```python
from build123d import *

# Parameters (mm, degrees)
SKETCH_1_W          = 8.99
SKETCH_1_H          = 1.99
EXTRUDE_1_DEPTH     = 1
EXTRUDE_2_DEPTH     = 8.99
SKETCH_3_W          = 1.62690844
SKETCH_3_H          = 0.234992706
CUT_EXTRUDE_2_DEPTH = 8.9
SKETCH_4_W          = 5.293711796
SKETCH_4_H          = 1.344910324
EXTRUDE_3_DEPTH     = 0.5
SKETCH_5_W          = 4.74668983
SKETCH_5_H          = 1.99
EXTRUDE_4_DEPTH     = 0.5
CHAMFER_1_SIZE      = 0.1
CHAMFER_2_SIZE      = 0.1


with BuildPart() as part:
    # 草图1 → 凸台-拉伸1 (new body)
    with BuildSketch(Plane(origin=(0, 0, 0), x_dir=(1, 0, 0), z_dir=(0, 1, 0))):
        Rectangle(SKETCH_1_W, SKETCH_1_H)
    extrude(amount=EXTRUDE_1_DEPTH)

    # 草图2 → 凸台-拉伸2 (add)
    with BuildSketch(Plane(origin=(4.495, 0, 0), x_dir=(0, 0, -1), z_dir=(1, 0, 0))):
        Polygon((-0.995, 0.5), (-1.355023595, 0.5), (-0.995, 1), align=None)
    extrude(amount=-EXTRUDE_2_DEPTH)

    # 草图3 → 切除-拉伸2 (cut)
    with BuildSketch(Plane(origin=(4.495, 0, 0), x_dir=(0, 0, -1), z_dir=(1, 0, 0))):
        with Locations((0, 0.75)):
            Rectangle(SKETCH_3_W, SKETCH_3_H)
    extrude(amount=-CUT_EXTRUDE_2_DEPTH, mode=Mode.SUBTRACT)

    # 草图4 → 凸台-拉伸3 (add)
    with BuildSketch(Plane.XZ):
        Rectangle(SKETCH_4_W, SKETCH_4_H)
    extrude(amount=EXTRUDE_3_DEPTH)

    # 草图5 → 凸台-拉伸4 (add)
    with BuildSketch(Plane(origin=(0, 1, 0), x_dir=(1, 0, 0), z_dir=(0, 1, 0))):
        Rectangle(SKETCH_5_W, SKETCH_5_H)
    extrude(amount=-EXTRUDE_4_DEPTH)

    # 倒角1
    chamfer_1_edges = [part.edges().sort_by_distance(p)[0] for p in [
        (2.646855898, 0, 0),
        (0, 0, 0.672455162),
        (-2.646855898, 0, 0),
        (0, 0, -0.672455162),
        (2.646855898, -0.5, 0),
        (0, -0.5, 0.672455162),
        (-2.646855898, -0.5, 0),
        (0, -0.5, -0.672455162),
        (0, 0, 0.995),
        (-4.495, 0, 0),
        (0, 0, -0.995),
        (4.495, 0, 0),
    ]]
    chamfer(chamfer_1_edges, length=CHAMFER_1_SIZE)

    # 倒角2
    chamfer_2_edges = [part.edges().sort_by_distance(p)[0] for p in [
        (0, 1, -0.995),
    ]]
    chamfer(chamfer_2_edges, length=CHAMFER_2_SIZE)


solid = part.part
```
Can you work these out from the model? Positions are in its coordinate system, mm. A direction names the side the tool comes from. Coordinates: 2 decimals unless noted, no trailing zeros. Loops run counter-clockwise (first coordinate to the right, second up) from the corner with the lowest first, then second, coordinate; pieces in that order, holes last. Notation, with made-up numbers: M 49.5,-13 L 89.5,-13 A23 ccw 89.5,1 Z; hole C 40.25,49.5 d8. An arc over 180 degrees is marked long. Put each result on its own line as item: value. Start each with the question number.
(1) I need wall thicknesses on probe 1 along Z at (x, y) = (-4, 0.15) (3 decimals); probe 2 along Z at (x, y) = (4.25, 0.8) (3 decimals); probe 3 along X at (y, z) = (-0.3, 0.55). Which ranges of each line are inside material? Lowest first, please.
(2) Imagine slicing it at D-D on z = 1.25. List the corners of the cut face in (x, y) for me (3 decimals).
(3) Will this pin go through, and if not, where does the flat tip stop? pin 1 Ø0.5 at (x, z) = (3.5, 0) entering from -Y.
(4) We'd pull the mould along Z, two halves only. Please class faces 3 (the face through (-3, 0.633, 0)), 4 (the face through (-4.495, 0.5, 0.2)): +Z half, -Z half, draft (parallel to the pull), parting line (faces both ways), or undercut.
(5) Imagine slicing it at C-C on x = 2.25. List the corners of the cut face in (y, z) for me (3 decimals).
(6) Which directions (+Z, -Z, +X, -X, +Y, -Y) give clear straight access to the entire face, cutting with the end or side of a thin tool? Please do faces 1 (the face through (4.495, 0.46, 0.16)), 2 (the face through (3, 0.633, 0)).
Worked answers:
1. probe 1: z = -0.995 to 0.995
1. probe 2: z = -0.995 to -0.813, 0.813 to 1.139
1. probe 3: x = -2.65 to 2.65
2. outline: M -4.495,0.5 L 4.495,0.5 L 4.495,0.646 L -4.495,0.646 Z
3. pin 1: stops at y = 0
4. face 3: undercut
4. face 4: draft
5. outline: M -0.5,-0.572 L -0.4,-0.672 L -0.1,-0.672 L 0,-0.772 L 0,-0.895 L 0.1,-0.995 L 0.9,-0.995 L 1,-0.895 L 1,0.995 L 0.5,1.355 L 0.5,0.995 L 0.1,0.995 L 0,0.895 L 0,0.772 L -0.1,0.672 L -0.4,0.672 L -0.5,0.572 Z
6. face 1: +Z, -Z, +X, +Y, -Y
6. face 2: +X
